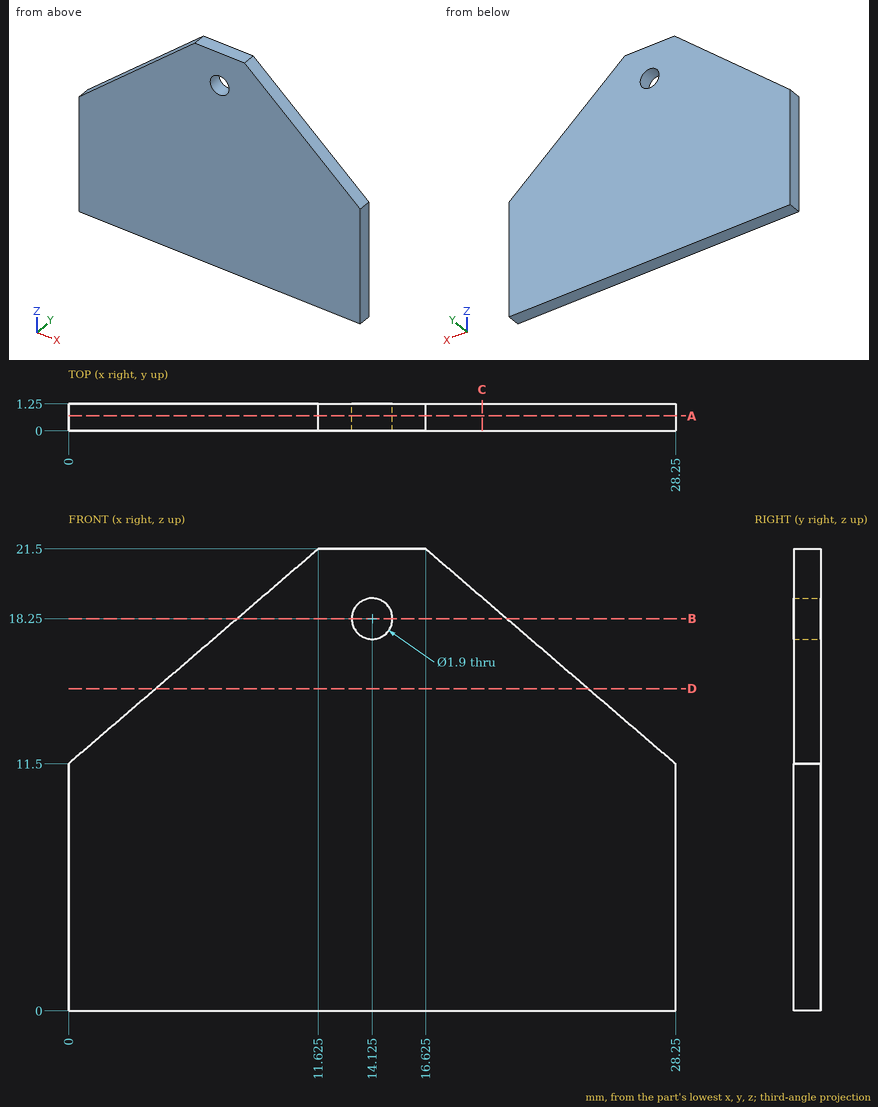
Can you work these out from the drawing? Everything is in mm from the part's minimum corner. Round coordinates to 2 decimals unless told otherwise and drop trailing zeros. Order: outer loops, then holes, each group sorted by start corner. A loop starts at its lowest first (then second) coordinate and runs counter-clockwise, first axis right, second up. Notation, with made-up numbers: (22.5, -12) -> (43.5, -12) arc R11 ccw to (43.5, 9) -> close; hole circle Ø2 at (37, -25.75). An arc over 180 degrees is marked (long way). Use CSV: the item, a comma, the result in double quotes.
1. I'm going to push flat-ended pins straight in: P1, Ø5, axis at x = 3.5, z = 17.5, coming from the +Y side; P2, Ø1.5, axis at x = 14.125, z = 18.25, coming from the -Y side. Where does each tip first touch, or does it pass through?
Recorded:
P1,"stops at y = 1.25"
P2,"passes through"
2. I want a section at B-B on z = 18.25. List the corners of the cut face in (x, y) for me (3 decimals), and give its area (3 significant figures).
Recorded:
outline,"(7.847, 0) -> (13.175, 0) -> (13.175, 1.25) -> (7.847, 1.25) -> close; (15.075, 0) -> (20.403, 0) -> (20.403, 1.25) -> (15.075, 1.25) -> close"
area,"13.3 mm2"
3. I want a section at C-C on x = 19.25. List the corners of the cut face in (y, z) for me, and give its area (3 significant figures).
Recorded:
outline,"(0, 0) -> (1.25, 0) -> (1.25, 19.24) -> (0, 19.24) -> close"
area,"24.1 mm2"
4. I want a section at A-A on y = 0.7. List the corners of the cut face in (x, z) for me (3 decimals), and give its area (3 significant figures).
Recorded:
outline,"(0, 0) -> (28.25, 0) -> (28.25, 11.5) -> (16.625, 21.5) -> (11.625, 21.5) -> (0, 11.5) -> close; hole circle Ø1.9 at (14.125, 18.25)"
area,"488 mm2"
5. I need wall thicknesses on line 1 along Z through (x, y) = (19.75, 0.7); line 2 along Z through (x, y) = (18, 1.2); line 3 along X through (y, z) = (0.2, 16.25). Which ranges of each line are inside material? Lowest first, please.
Recorded:
line 1,"z = 0 to 18.81"
line 2,"z = 0 to 20.32"
line 3,"x = 5.52 to 22.73"
6. I want a section at D-D on z = 15. List the corners of the cut face in (x, y) for me, and give its area (3 significant figures).
Recorded:
outline,"(4.07, 0) -> (24.18, 0) -> (24.18, 1.25) -> (4.07, 1.25) -> close"
area,"25.1 mm2"
